Input: part model. Units: mm. Frame: model coordinates. A direction names the side the tool comes from. Give positions to 0.01 mm unless a question says otherwise; leave off trailing zeros. Write each loop counter-clockwise with the first axis right and the second up, starting at its lowest first coordinate (ties: lowest second). Pieces come first, ordered by that corner, then holes. Notation, with made-up numbers: (59.25, 50.25) - (94.25, 50.25) arc R14 ccw to (94.25, 61.25) - close; hole circle Ø4 at (-1, 11). An arc over 180 degrees is marked (long way). Answer as a JSON object with one key per item and string values. Group by question number.
from build123d import *

# Parameters (mm, degrees)
SKETCH1_W           = 211.1375
SKETCH1_H           = 35.56
BOSS_EXTRUDE1_DEPTH = 9.525
SKETCH6_R           = 12.192
BOSS_EXTRUDE4_DEPTH = 6.35
BOSS_EXTRUDE5_DEPTH = 3.175
LPATTERN1_COUNT     = 22
LPATTERN1_PITCH     = 9.525
SKETCH10_W          = 59.980257814
SKETCH10_H          = 67.271975432
CUT_EXTRUDE1_DEPTH  = 125.4125
SKETCH11_W          = 24.384
SKETCH11_H          = 7.0104
BOSS_EXTRUDE6_DEPTH = 12.7


with BuildPart() as part:
    # Sketch1 → Boss-Extrude1 (new body)
    with BuildSketch(Plane(origin=(0, 0, 0), x_dir=(1, 0, 0), z_dir=(0, 1, 0))):
        with Locations((-105.56875, 17.78)):
            Rectangle(SKETCH1_W, SKETCH1_H)
    extrude(amount=BOSS_EXTRUDE1_DEPTH)

    # Sketch6 → Boss-Extrude4 (add)
    with BuildSketch(Plane(origin=(0, 0, 0), x_dir=(-1, 0, 0), z_dir=(0, -1, 0))):
        with Locations((105.56875, 17.78)):
            Circle(SKETCH6_R)
        with Locations((36.79825, 17.78)):
            Circle(SKETCH6_R)
        with Locations((174.33925, 17.78)):
            Circle(SKETCH6_R)
    extrude(amount=BOSS_EXTRUDE4_DEPTH)

    # Sketch9 → Boss-Extrude5 (add)
    with BuildSketch(Plane.ZY.offset(204.7875)):
        Polygon((-35.56, 9.525), (0, 9.525), (-8.89, 34.417), align=None)
    boss_extrude5 = extrude(amount=-BOSS_EXTRUDE5_DEPTH)

    # LPattern1: Boss-Extrude5 ×22
    with Locations(*[(i * LPATTERN1_PITCH, 0, 0) for i in range(1, LPATTERN1_COUNT)]):
        add(boss_extrude5)

    # Sketch10 → Cut-Extrude1 (cut)
    with BuildSketch(Plane(origin=(0, 0, 0), x_dir=(0, 0, -1), z_dir=(1, 0, 0))):
        with Locations((17.78, 4.683648782)):
            Rectangle(SKETCH10_W, SKETCH10_H)
    extrude(amount=-CUT_EXTRUDE1_DEPTH, mode=Mode.SUBTRACT)

    # Sketch11 → Boss-Extrude6 (add)
    with BuildSketch(Plane(origin=(-125.4125, 0, 0), x_dir=(0, 0, -1), z_dir=(1, 0, 0))):
        with Locations((17.78, 4.7625)):
            Rectangle(SKETCH11_W, SKETCH11_H)
    extrude(amount=BOSS_EXTRUDE6_DEPTH)


solid = part.part
1) Reachability of faces 1 (the face through (-138.112, 17, -14)), 2 (the face through (-119, 8.268, -18)), 3 (the face through (-165.122, 21.797, -4.383)) from +Z, -Z, +X, -X, +Y, -Y: full face, straight path, thin tool, end or side. Return the list, or none.
2) Mould query, pull axis X, two halves, no side actions, for faces 4 (the face through (-119, 5, -29.972)), 5 (the face through (-112.712, 5, -18)), 6 (the face through (-182.562, 17, -14)). Classes: +X half, -X half, draft (parallel to the pull), parting line (faces both ways), or undercut.
3) Cut plane A-A on x = -127. Return the cut outline in (y, z) (3 decimals), and give its area (3 significant figures).
4) Pin query (flat end, axial travel): P1, Ø20, axis at y = 24, z = -10, coming from the +X side; P2, Ø8, axis at x = -152.5, z = -7, coming from the -Y side; P3, Ø6.5, axis at x = -116, z = -22.5, coming from the +Y side. Return the tip coordinate at first contact, or that it passes through.
5) Line query: line 1 along Y through (x, z) = (-132, -23) (3 decimals); line 2 along Y through (x, z) = (-177.5, -22) (3 decimals); line 3 along X through (y, z) = (-2, -15.5). Output: solid intervals per line, ascending. Write a range as from..to.
6) Cut plane B-B on y = 14. Count the separate pieces of the cut face and the enclosed holes in it, and give its area (3 significant figures).
Filled in:
{
 "1": {"face 1": "+Z, -Z, +Y", "face 2": "+Z, -Z, +X, +Y", "face 3": "+Z, +X, -X, +Y"},
 "2": {"face 4": "draft", "face 5": "+X half", "face 6": "undercut"},
 "3": {"outline": "(0, -35.56) - (9.525, -35.56) - (34.417, -8.89) - (9.525, 0) - (0, 0) - close", "area": "781 mm²"},
 "4": {"P1": "stops at x = -125.41", "P2": "stops at y = 0", "P3": "stops at y = 8.27"},
 "5": {"line 1": "y = 0..9.525", "line 2": "y = -6.35..9.525", "line 3": "x = -186.32..-162.36"},
 "6": {"separate pieces": "9", "enclosed holes": "0", "area": "833 mm²"}
}
